Build history of the part. All positions in model axes, mm. A direction names the side the tool comes from. Give positions to 0.01 mm unless a question says otherwise; leave off trailing zeros. Write each loop counter-clockwise with the first axis right and the second up, starting at its lowest first coordinate (ties: lowest second). Pieces come first, ordered by that corner, then holes. Notation, with made-up numbers: (4.25, -16) -> (49.25, -16) arc R18 ccw to (49.25, 12) -> close; hole circle Ø4 at (-23, 45). An arc over 180 degrees is marked (long way). Put each result on its own line as item: value. Start each with the question number.
Item 1: Drill centre lines: line 1 along X through (y, z) = (-365, -173); line 2 along Y through (x, z) = (0, -165); line 3 along Y through (x, z) = (2, -66.5). Where is each one in solid material? Low to high.
Item 2: Tool access for faces 4 (the flat face through (-195, -345, -37)), 5 (the flat face through (0, -350, -77)), 6 (the flat face through (-15, -158, 0)): list every direction of +Z, -Z, +X, -X, +Y, -Y with a clear straight run to the whole face (end or side of a thin tool).
Item 3: Slice it at B-B, the plane y = -25. List the corners of the cut face in (x, z), plus the area to 3 significant figures.
Item 4: Slice it at D-D, the plane x = -127.5. List the corners of the cut face in (y, z), plus the area to 3 significant figures.
Item 5: Slice it at C-C, the plane z = -31. List the corners of the cut face in (x, y).
Item 6: Two-plate mould, pull along X, no slides. Class faces 1 (the flat face through (0, -525, -77)), 2 (the flat face through (-180, -360, -66)), 3 (the flat face through (15, -320, -7)): pulls with the +X half, pulls with the -X half, needs draft (parallel to the pull), parting line crosses it, or undercut.
Item 7: Slice it at A-A, the plane z = -171. List the corners of the cut face in (x, y), plus the area to 3 significant figures.
Item 8: Flat gauge pins, fed straight in: pin 1 Ø15 at (x, y) = (4.5, -454) entering from -Z; pin 2 Ø20 at (x, y) = (-197.5, -330) entering from -Z; pin 3 Ø12 at (x, z) = (-141.5, -20.5) entering from +Y; pin 4 Ø4 at (x, z) = (-212.5, -0.5) entering from -Y. Where does each tip first touch, or does it go through?
```python
from build123d import *

# Parameters (mm, degrees)
F0_W      = 30
F0_H      = 25
F1_DEPTH  = 560
F2_W      = 30
F2_H      = 25
F3_DEPTH  = 200
F4_R      = 10
F5_DEPTH  = 25
F6_W      = 30
F6_H      = 30
F7_DEPTH  = 130
F8_SIZE   = 5
F9_R      = 7.5
F9_R_2    = 4
F10_DEPTH = 50
F12_R     = 7.5
F12_R_2   = 4
F13_DEPTH = 50
F14_W     = 30
F14_H     = 30
F15_DEPTH = 5
F16_W     = 30
F16_H     = 5
F17_DEPTH = 40
F18_W     = 30
F18_H     = 130
F19_DEPTH = 30
F20_SIZE  = 5
F21_R     = 7.5
F21_R_2   = 4
F22_DEPTH = 50
F23_W     = 30
F23_H     = 5
F24_DEPTH = 25


# Not quite as in the source:
# - two fillets or chamfers of one size are made in one step


with BuildPart() as f1:
    # F0 (on Front) → F1 (new body)
    with BuildSketch(Plane.XZ):
        Rectangle(F0_W, F0_H)
    extrude(amount=F1_DEPTH)

    # F2 (on face) → F3 (join)
    with BuildSketch(Plane(origin=(-15, 0, 0), x_dir=(0, -1, 0), z_dir=(-1, 0, 0))):
        with Locations((335, 0)):
            Rectangle(F2_W, F2_H)
    extrude(amount=F3_DEPTH)

    # F4 (on face) → F5 (cut)
    with BuildSketch(Plane.XY.offset(12.5)):
        with Locations((0, -25)):
            Circle(F4_R)
    extrude(amount=-F5_DEPTH, mode=Mode.SUBTRACT)

    # F6 (on face) → F7 (join)
    with BuildSketch(Plane(origin=(0, 0, -12.5), x_dir=(1, 0, 0), z_dir=(0, 0, -1))):
        with Locations((0, 540)):
            Rectangle(F6_W, F6_H)
        with Locations((0, 365)):
            Rectangle(F6_W, F6_H)
    extrude(amount=F7_DEPTH)

    # F8
    f8_edges = [f1.edges().sort_by_distance(p)[0] for p in [
        (-15, -555, -77.5),
        (15, -555, -77.5),
        (15, -525, -77.5),
        (-15, -525, -77.5),
        (15, -350, -77.5),
        (15, -380, -77.5),
        (-15, -350, -77.5),
        (-15, -380, -77.5),
    ]]
    chamfer(f8_edges, length=F8_SIZE)

    # F9 (on face) → F10 (join)
    with BuildSketch(Plane(origin=(0, 0, -142.5), x_dir=(1, 0, 0), z_dir=(0, 0, -1))):
        with Locations((0, 540)):
            Circle(F9_R)
        with Locations((0, 540)):
            Circle(F9_R_2, mode=Mode.SUBTRACT)
    extrude(amount=F10_DEPTH)

    # F12 (on face) → F13 (join)
    with BuildSketch(Plane(origin=(0, 0, -142.5), x_dir=(1, 0, 0), z_dir=(0, 0, -1))):
        with Locations((0, 365)):
            Circle(F12_R)
        with Locations((0, 365)):
            Circle(F12_R_2, mode=Mode.SUBTRACT)
    extrude(amount=F13_DEPTH)

    # F14 (on face) → F15 (join)
    with BuildSketch(Plane(origin=(0, 0, -12.5), x_dir=(1, 0, 0), z_dir=(0, 0, -1))):
        with Locations((-195, 335)):
            Rectangle(F14_W, F14_H)
    extrude(amount=F15_DEPTH)

    # F16 (on face) → F17 (join)
    with BuildSketch(Plane(origin=(0, 0, -17.5), x_dir=(1, 0, 0), z_dir=(0, 0, -1))):
        with Locations((-195, 347.5)):
            Rectangle(F16_W, F16_H)
    extrude(amount=F17_DEPTH)

    # F18 (on face) → F19 (join)
    with BuildSketch(Plane.XZ.offset(350)):
        with Locations((-195, -77.5)):
            Rectangle(F18_W, F18_H)
    extrude(amount=F19_DEPTH)

    # F20
    f20_edges = [f1.edges().sort_by_distance(p)[0] for p in [
        (-210, -380, -77.5),
        (-180, -380, -77.5),
        (-180, -350, -100),
        (-210, -350, -100),
    ]]
    chamfer(f20_edges, length=F20_SIZE)

    # F21 (on face) → F22 (join)
    with BuildSketch(Plane(origin=(0, 0, -142.5), x_dir=(1, 0, 0), z_dir=(0, 0, -1))):
        with Locations((-195, 365)):
            Circle(F21_R)
        with Locations((-195, 365)):
            Circle(F21_R_2, mode=Mode.SUBTRACT)
    extrude(amount=F22_DEPTH)

    # F23 (on face) → F24 (join)
    with BuildSketch(Plane.XY.offset(-12.5)):
        with Locations((-195, -352.5)):
            Rectangle(F23_W, F23_H)
    extrude(amount=F24_DEPTH)


solid = f1.part
```
Values follow:
1. line 1: -202.5 to -199, -191 to -187.5, -7.5 to -4, 4 to 7.5
1. line 2: -547.5 to -544, -536 to -532.5, -372.5 to -369, -361 to -357.5
1. line 3: -555 to -525, -380 to -350
2. face 4: -Z, +X, -X, +Y
2. face 5: -Z, +X, +Y
2. face 6: +Z, -Z, -X, +Y
3. outline: (-15, -12.5) -> (-10, -12.5) -> (-10, 12.5) -> (-15, 12.5) -> close; (10, -12.5) -> (15, -12.5) -> (15, 12.5) -> (10, 12.5) -> close
3. area: 250 mm2
4. outline: (-350, -12.5) -> (-320, -12.5) -> (-320, 12.5) -> (-350, 12.5) -> close
4. area: 750 mm2
5. outline: (-210, -375) -> (-205, -380) -> (-185, -380) -> (-180, -375) -> (-180, -345) -> (-210, -345) -> close; (-15, -550) -> (-10, -555) -> (10, -555) -> (15, -550) -> (15, -530) -> (10, -525) -> (-10, -525) -> (-15, -530) -> close; (-15, -375) -> (-10, -380) -> (10, -380) -> (15, -375) -> (15, -355) -> (10, -350) -> (-10, -350) -> (-15, -355) -> close
6. face 1: needs draft
6. face 2: undercut
6. face 3: pulls with the +X half
7. outline: circle Ø15 at (-195, -365); circle Ø15 at (0, -540); circle Ø15 at (0, -365); hole circle Ø8 at (-195, -365); hole circle Ø8 at (0, -540); hole circle Ø8 at (0, -365)
7. area: 379 mm2
8. pin 1: z = -12.5
8. pin 2: z = -17.5
8. pin 3: through
8. pin 4: y = -350
